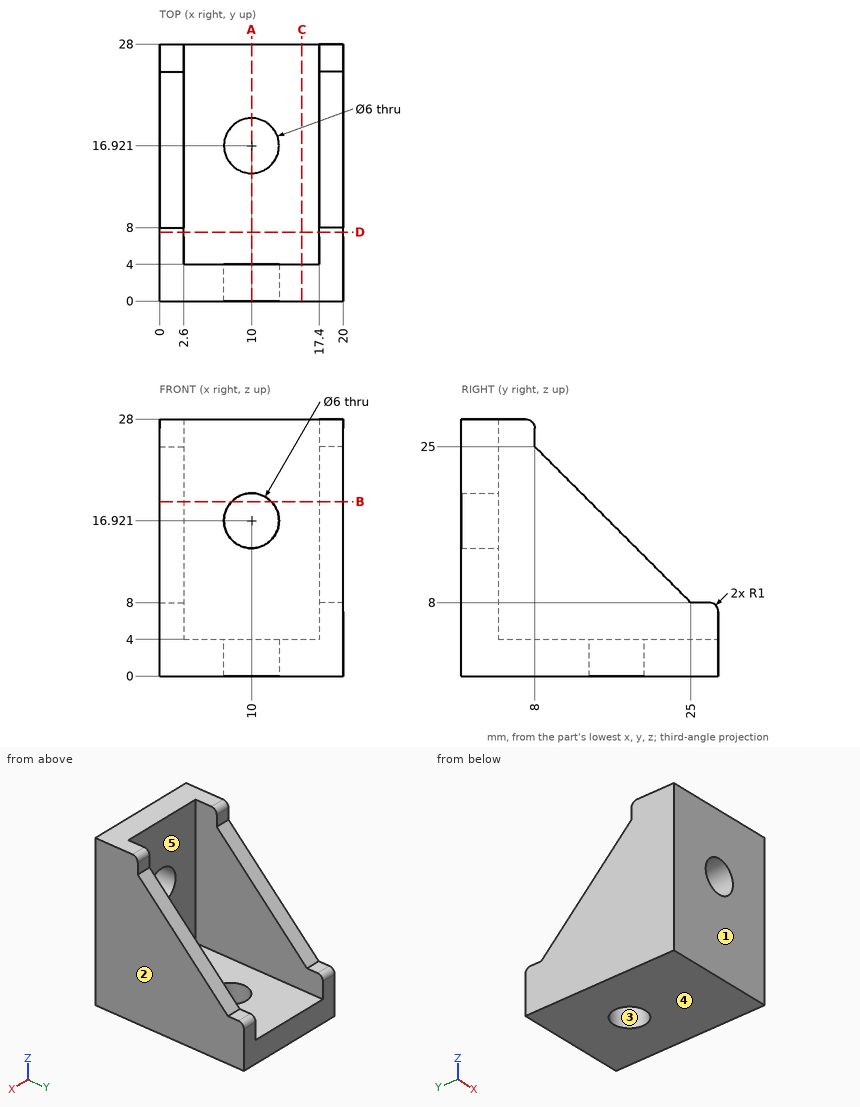
Part print with two shaded views. Sizes in mm from the minimum x, y, z corner. A direction names the side the tool comes from. Round coordinates to 2 decimals unless told otherwise and drop trailing zeros. Order: outer loops, then holes, each group sorted by start corner. A loop starts at its lowest first (then second) coordinate and runs counter-clockwise, first axis right, second up. Notation, with made-up numbers: (0, 40.25) - (23, 40.25) arc R15 cw to (23, 64.25) - close; hole circle Ø8 at (33, 47). An arc over 180 degrees is marked (long way). Answer as CSV lines item,"result". Start each with the question number.
1. Saw through at B-B, the plane z = 19. Write the cut outline in (x, y), and give its area (3 significant figures).
2. Saw through at D-D, the plane y = 7.5. Write the cut outline in (x, z), and give its area (3 significant figures).
3. Saw through at A-A, the plane x = 10. Write the cut outline in (y, z).
4. Drill centre lines: L1, parallel to Z at x = 10, y = 2.2; L2, parallel to X at y = 6, z = 6.5; L3, parallel to Y at x = 16.5, z = 4.5. Where is each one in solid material? Low to high. Write a range as [from, to].
5. Tool access for the marked faces 4 and 5: list every direction of +Z, -Z, +X, -X, +Y, -Y with a clear straight run to the whole face (end or side of a thin tool).
6. Pin check, flat tips, straight feed: pin 1 (8 mm diameter, centred on x = 10, z = 16.92, fed in from -Y); pin 2 (8 mm diameter, centred on x = 10, y = 16.92, fed in from +Z); pin 3 (1.6 mm diameter, centred on x = 1, z = 25.5, fed in from +Y); pin 4 (1 mm diameter, centred on x = 11.5, z = 20.5, fed in from +Y). Stop position of each tip, or through.
7. Pull direction Y, two halves, no side cores. Call the marked faces 1, 2 and 3: +Y half, -Y half, draft (parallel to the pull), parting line (faces both ways), or undercut.
8. Saw through at C-C, the plane x = 15.5. Write the cut outline in (y, z), and give its area (3 significant figures).
Model answer:
1,outline,"(0, 0) - (7.84, 0) - (7.84, 4) - (2.6, 4) - (2.6, 14) - (0, 14) - close; (12.16, 0) - (20, 0) - (20, 14) - (17.4, 14) - (17.4, 4) - (12.16, 4) - close"
1,area,"115 mm²"
2,outline,"(0, 0) - (20, 0) - (20, 27.87) - (17.4, 27.87) - (17.4, 4) - (2.6, 4) - (2.6, 27.87) - (0, 27.87) - close"
2,area,"204 mm²"
3,outline,"(0, 0) - (13.92, 0) - (13.92, 4) - (4, 4) - (4, 13.92) - (0, 13.92) - close; (0, 19.92) - (4, 19.92) - (4, 28) - (0, 28) - close; (19.92, 0) - (28, 0) - (28, 4) - (19.92, 4) - close"
4,L1,"z = [0, 13.92], [19.92, 28]"
4,L2,"x = [0, 2.6], [17.4, 20]"
4,L3,"y = [0, 4]"
5,face 4,"-Z, +X, -X, +Y, -Y"
5,face 5,"+Z, +Y"
6,pin 1,"stops at y = 0"
6,pin 2,"stops at z = 4"
6,pin 3,"stops at y = 8.3"
6,pin 4,"stops at y = 4"
7,face 1,"-Y half"
7,face 2,"draft"
7,face 3,"undercut"
8,outline,"(0, 0) - (28, 0) - (28, 4) - (4, 4) - (4, 28) - (0, 28) - close"
8,area,"208 mm²"
